```python
from build123d import *

# Parameters (mm, degrees)
SKETCH2_W           = 101.6
SKETCH2_H           = 25.4
BOSS_EXTRUDE1_DEPTH = 25.4
SKETCH3_W           = 101.6
SKETCH3_H           = 19.05
CUT_EXTRUDE1_DEPTH  = 22.225
CUT_EXTRUDE2_DEPTH  = 25.4
CUT_EXTRUDE3_DEPTH  = 25.4
SKETCH6_R           = 1.524
CUT_EXTRUDE4_DEPTH  = 3.175
SKETCH7_R           = 1.524
CUT_EXTRUDE5_DEPTH  = 3.175
FILLET1_R           = 3.048
FILLET2_R           = 3.048
FILLET3_R           = 3.048


with BuildPart() as part:
    # Sketch2 → Boss-Extrude1 (new body)
    with BuildSketch(Plane(origin=(0, 25.4, 0), x_dir=(1, 0, 0), z_dir=(0, 1, 0))):
        with Locations((25.998060942, 0.45734072)):
            Rectangle(SKETCH2_W, SKETCH2_H)
    extrude(amount=BOSS_EXTRUDE1_DEPTH)

    # Sketch3 → Cut-Extrude1 (cut)
    with BuildSketch(Plane.XY.offset(12.24265928)):
        with Locations((25.998060942, 38.1)):
            Rectangle(SKETCH3_W, SKETCH3_H)
    extrude(amount=-CUT_EXTRUDE1_DEPTH, mode=Mode.SUBTRACT)

    # Sketch4 → Cut-Extrude2 (cut)
    with BuildSketch(Plane(origin=(0, 50.8, 0), x_dir=(1, 0, 0), z_dir=(0, 1, 0))):
        with BuildLine():
            Line((-13.689439058, 0.39384072), (24.220060942, 0.39384072))
            ThreePointArc((24.220060942, 0.39384072), (25.744060942, -1.13015928), (24.220060942, -2.65415928))
            Line((24.220060942, -2.65415928), (-13.689439058, -2.65415928))
            ThreePointArc((-13.689439058, -2.65415928), (-15.213439058, -1.13015928), (-13.689439058, 0.39384072))
        make_face()
    extrude(amount=-CUT_EXTRUDE2_DEPTH, mode=Mode.SUBTRACT)

    # Sketch5 → Cut-Extrude3 (cut)
    with BuildSketch(Plane(origin=(0, 50.8, 0), x_dir=(1, 0, 0), z_dir=(0, 1, 0))):
        with BuildLine():
            Line((27.776060942, 0.39384072), (65.685560942, 0.39384072))
            ThreePointArc((65.685560942, 0.39384072), (67.209560942, -1.13015928), (65.685560942, -2.65415928))
            Line((65.685560942, -2.65415928), (27.776060942, -2.65415928))
            ThreePointArc((27.776060942, -2.65415928), (26.252060942, -1.13015928), (27.776060942, 0.39384072))
        make_face()
    extrude(amount=-CUT_EXTRUDE3_DEPTH, mode=Mode.SUBTRACT)

    # Sketch6 → Cut-Extrude4 (cut)
    with BuildSketch(Plane(origin=(0, 50.8, 0), x_dir=(1, 0, 0), z_dir=(0, 1, 0))):
        with Locations(Location((5.265310942, -7.44840928, 0), (0, 0, 270))):
            Circle(SKETCH6_R)
        with Locations(Location((5.265310942, 5.18809072, 0), (0, 0, 270))):
            Circle(SKETCH6_R)
        with Locations(Location((46.730810942, 5.18809072, 0), (0, 0, 270))):
            Circle(SKETCH6_R)
        with Locations(Location((46.730810942, -7.44840928, 0), (0, 0, 270))):
            Circle(SKETCH6_R)
    extrude(amount=-CUT_EXTRUDE4_DEPTH, mode=Mode.SUBTRACT)

    # Sketch7 → Cut-Extrude5 (cut)
    with BuildSketch(Plane(origin=(0, 0, -13.15734072), x_dir=(-1, 0, 0), z_dir=(0, 0, -1))):
        with Locations((-56.478060942, 38.1)):
            Circle(SKETCH7_R)
        with Locations((-36.158060942, 38.1)):
            Circle(SKETCH7_R)
        with Locations((-15.838060942, 38.1)):
            Circle(SKETCH7_R)
        with Locations((4.481939058, 38.1)):
            Circle(SKETCH7_R)
    extrude(amount=-CUT_EXTRUDE5_DEPTH, mode=Mode.SUBTRACT)

    # Fillet1
    fillet1_edges = [part.edges().sort_by_distance(p)[0] for p in [
        (25.998060942, 47.625, -9.98234072),
        (25.998060942, 28.575, -9.98234072),
    ]]
    fillet(fillet1_edges, radius=FILLET1_R)

    # Fillet2
    fillet2_edges = [part.edges().sort_by_distance(p)[0] for p in [
        (25.998060942, 50.8, -13.15734072),
        (25.998060942, 25.4, -13.15734072),
    ]]
    fillet(fillet2_edges, radius=FILLET2_R)

    # Fillet3
    fillet3_edges = [part.edges().sort_by_distance(p)[0] for p in [
        (76.798060942, 26.9875, 12.24265928),
        (-24.801939058, 26.9875, 12.24265928),
        (76.798060942, 49.2125, 12.24265928),
        (-24.801939058, 49.2125, 12.24265928),
    ]]
    fillet(fillet3_edges, radius=FILLET3_R)


solid = part.part
```
Work out the finished part from the listing and answer in its coordinate system (mm). A direction names the side the tool comes from. Give positions to 0.01 mm unless a question says otherwise; leave off trailing zeros. Write each loop counter-clockwise with the first axis right and the second up, starting at its lowest first coordinate (ties: lowest second). Pieces come first, ordered by that corner, then holes. Notation, with made-up numbers: (89, 15.25) -> (100, 15.25) arc R11 ccw to (100, 29.25) -> close; hole circle Ø7 at (-12.75, -5). An arc over 180 degrees is marked (long way). Write item = value, one per line.
Q1. Flat-ended cylindrical pins translate along their axes: pin 1 Ø1.6 at (x, y) = (-2.5, 49.5) entering from -Z; pin 2 Ø4 at (x, y) = (36.16, 38.1) entering from -Z; pin 3 Ø10.5 at (x, y) = (38, 38) entering from +Z. Find the tip coordinate at first contact, or state that the pin passes through.
Computed values:
pin_1 = -13.01
pin_2 = -13.16
pin_3 = -9.98
Q2. For a pull along Y with two mould halves and no side action, classify faces 4 (the cylindrical face through (26.71, 49.93, -12.24)), 5 (the cylindrical face through (-5.301, 39.385, -11.592)), 6 (the cylindrical face through (-15.213, 27.01, 1.164)), 7 (the flat face through (25, 25.4, -2)) as pulls with the +Y half, pulls with the -Y half, needs draft (parallel to the pull), parting line crosses it, or undercut.
Computed values:
face_4 = pulls with the +Y half
face_5 = undercut
face_6 = needs draft
face_7 = pulls with the -Y half
Q3. A tool of negligible diameter and unlimited length cuts with its end or side. For faces 1 (the cylindrical face through (58, 38, -12)), 2 (the cylindrical face through (4.338, 49.235, 6.239)), 3 (the cylindrical face through (25.744, 27.01, 1.097)), from which of +Z, -Z, +X, -X, +Y, -Y can it reach the whole face along a straight path? Write none if from no direction.
Computed values:
face_1 = +Z, -Z
face_2 = +Y
face_3 = +Y, -Y
Q4. Section A-A on y = 38.1 is taken. Determine the outline of the cut face in (x, z), and give its area (3 significant figures).
Computed values:
outline = (-24.8, -13.16) -> (-6.01, -13.16) -> (-6.01, -9.98) -> (-24.8, -9.98) -> close; (-2.96, -13.16) -> (14.31, -13.16) -> (14.31, -9.98) -> (-2.96, -9.98) -> close; (17.36, -13.16) -> (34.63, -13.16) -> (34.63, -9.98) -> (17.36, -9.98) -> close; (37.68, -13.16) -> (54.95, -13.16) -> (54.95, -9.98) -> (37.68, -9.98) -> close; (58, -13.16) -> (76.8, -13.16) -> (76.8, -9.98) -> (58, -9.98) -> close
area = 284 mm^2
Q5. Consider line 1 along Y through (x, z) = (50.5, -6.5) (3 decimals); line 2 along X through (y, z) = (48.75, 0.5); line 3 along Z through (x, y) = (12, 42.25). Determine where each line is inside the solid, lowest interval first.
Computed values:
line_1 = 25.4 to 28.575, 47.625 to 50.8
line_2 = -24.8 to -15.08, 25.61 to 26.39, 67.07 to 76.8
line_3 = -13.16 to -9.98
Q6. Section B-B on x = 19 is taken. Determine the outline of the cut face in (y, z) (3 decimals), and give its area (3 significant figures).
Computed values:
outline = (25.4, -10.109) arc R3.048 ccw to (28.448, -13.157) -> (47.752, -13.157) arc R3.048 ccw to (50.8, -10.109) -> (50.8, -0.394) -> (47.625, -0.394) -> (47.625, -6.934) arc R3.048 cw to (44.577, -9.982) -> (31.623, -9.982) arc R3.048 cw to (28.575, -6.934) -> (28.575, -0.394) -> (25.4, -0.394) -> close; (25.4, 2.654) -> (28.575, 2.654) -> (28.575, 12.243) -> (25.4, 12.243) -> close; (47.625, 2.654) -> (50.8, 2.654) -> (50.8, 12.243) -> (47.625, 12.243) -> close
area = 202 mm^2
Q7. Section C-C on z = 10.75 is taken. Determine the outline of the cut face in (x, y) (3 decimals), and give its area (3 significant figures).
Computed values:
outline = (-24.375, 25.4) -> (76.371, 25.4) -> (76.371, 28.575) -> (-24.375, 28.575) -> close; (-24.375, 47.625) -> (76.371, 47.625) -> (76.371, 50.8) -> (-24.375, 50.8) -> close
area = 640 mm^2
Q8. Section D-D on x = 68.5 is taken. Determine the outline of the cut face in (y, z) (3 decimals), and give its area (3 significant figures).
Computed values:
outline = (25.4, -10.109) arc R3.048 ccw to (28.448, -13.157) -> (47.752, -13.157) arc R3.048 ccw to (50.8, -10.109) -> (50.8, 12.243) -> (47.625, 12.243) -> (47.625, -6.934) arc R3.048 cw to (44.577, -9.982) -> (31.623, -9.982) arc R3.048 cw to (28.575, -6.934) -> (28.575, 12.243) -> (25.4, 12.243) -> close
area = 222 mm^2
